Source: three-view drawing plus pictorial views. Frame: mm from the lowest corner of the part. Give positions to 0.01 mm unless a question says otherwise; leave off trailing zeros. Order: outer loops, then holes, each group sorted by start corner. A loop starts at its lowest first (then second) coordinate and runs counter-clockwise, first axis right, second up. Notation, with made-up numbers: M -34.5,-33.5 L 9.5,-33.5 A9 cw 9.5,-28.5 Z; hole C 86,-28.75 d9. An arc over 180 degrees is marked long. Use CSV: the item, a comma, the result in double quotes. Start each with the question number.
1. Pin query (flat end, axial travel): P1, Ø5.5, axis at x = 20.75, z = 64.67, coming from the +Y side. Return the tip coordinate at first contact, or that it passes through.
2. Line query: line 1 along X through (y, z) = (10.5, 38.5); line 2 along Z through (x, y) = (45.5, 16); line 3 along X through (y, z) = (36.5, 64.5) (1 decimal). Output: solid intervals per line, ascending. Write a range as [from, to].
3. Section query D-D, the plane y = 26.5. Return the cut outline in (x, z) (1 decimal), plus the area to 3 significant figures.
4. Section query B-B, the plane z = 30. Return the cut outline in (x, y) (1 decimal).
5. Mould query, pull axis Z, two halves, no side actions, for the marked faces 1, 2 and 3. Classes: released by +Z, released by -Z, zero draft, split by the parting line, or undercut.
6. Section query A-A, the plane x = 39.5. Return the cut outline in (y, z) (1 decimal).
7. Section query C-C, the plane x = 23. Return the cut outline in (y, z), plus the area to 3 significant figures.
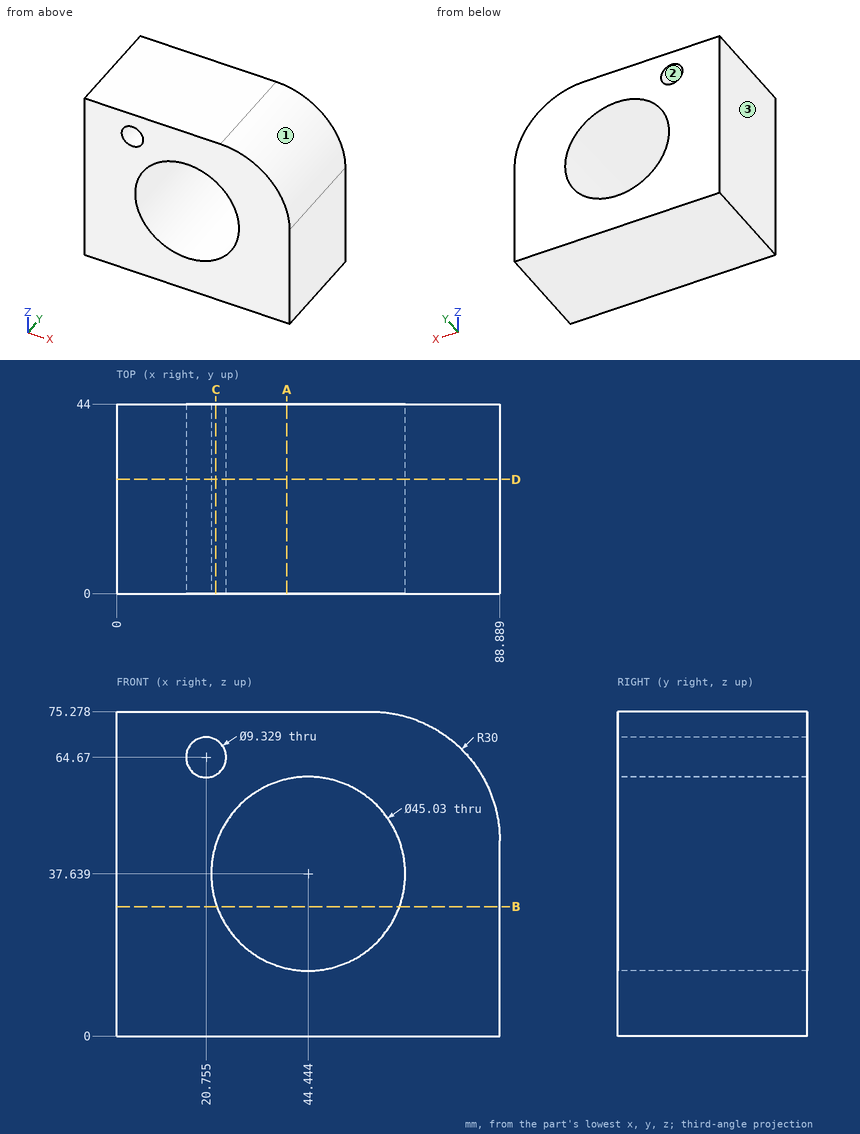
Result set:
1,P1,"through"
2,line 1,"[0, 21.95], [66.94, 88.89]"
2,line 2,"[0, 15.15], [60.13, 75.28]"
2,line 3,"[0, 16.1], [25.4, 81.9]"
3,outline,"M 0,0 L 88.9,0 L 88.9,45.3 A30 ccw 58.9,75.3 L 0,75.3 Z; hole C 20.8,64.7 d9.3; hole C 44.4,37.6 d45"
3,area,"4,840 mm2"
4,outline,"M 0,0 L 23.3,0 L 23.3,44 L 0,44 Z; M 65.6,0 L 88.9,0 L 88.9,44 L 65.6,44 Z"
5,face 1,"released by +Z"
5,face 2,"undercut"
5,face 3,"zero draft"
6,outline,"M 0,0 L 44,0 L 44,15.7 L 0,15.7 Z; M 0,59.6 L 44,59.6 L 44,75.3 L 0,75.3 Z"
7,outline,"M 0,0 L 44,0 L 44,30.78 L 0,30.78 Z; M 0,44.5 L 44,44.5 L 44,60.58 L 0,60.58 Z; M 0,68.76 L 44,68.76 L 44,75.28 L 0,75.28 Z"
7,area,"2,350 mm2"
